```python
from build123d import *

# Parameters (mm, degrees)
BOSS_EXTRUDE1_DEPTH = 2
CUT_EXTRUDE1_DEPTH  = 10


with BuildPart() as part:
    # Sketch1 → Boss-Extrude1 (new body)
    with BuildSketch(Plane.XY):
        with BuildLine():
            Line((-26.516504294, 44.194173824), (-44.194173824, 26.516504294))
            ThreePointArc((-44.194173824, 26.516504294), (-36.270318491, 0), (-44.194173824, -26.516504294))
            Line((-44.194173824, -26.516504294), (-26.516504294, -44.194173824))
            ThreePointArc((-26.516504294, -44.194173824), (0, -36.270318491), (26.516504294, -44.194173824))
            Line((26.516504294, -44.194173824), (44.194173824, -26.516504294))
            ThreePointArc((44.194173824, -26.516504294), (36.270318491, 0), (44.194173824, 26.516504294))
            Line((44.194173824, 26.516504294), (26.516504294, 44.194173824))
            ThreePointArc((26.516504294, 44.194173824), (0, 36.270318491), (-26.516504294, 44.194173824))
        make_face()
    extrude(amount=BOSS_EXTRUDE1_DEPTH)

    # Sketch2 → Cut-Extrude1 (cut)
    with BuildSketch(Plane(origin=(0, 0, 0), x_dir=(-1, 0, 0), z_dir=(0, 0, -1))):
        with BuildLine():
            Line((-27.708756501, -8.757507261), (-27.708756501, 8.757507261))
            ThreePointArc((-27.708756501, 8.757507261), (-22.708756501, 13.757507261), (-17.708756501, 8.757507261))
            Line((-17.708756501, 8.757507261), (-17.708756501, -8.757507261))
            ThreePointArc((-17.708756501, -8.757507261), (-22.708756501, -13.757507261), (-27.708756501, -8.757507261))
        make_face()
        with BuildLine():
            Line((27.708756501, -8.757507261), (27.708756501, 8.757507261))
            ThreePointArc((27.708756501, 8.757507261), (22.708756501, 13.757507261), (17.708756501, 8.757507261))
            Line((17.708756501, 8.757507261), (17.708756501, -8.757507261))
            ThreePointArc((17.708756501, -8.757507261), (22.708756501, -13.757507261), (27.708756501, -8.757507261))
        make_face()
        with BuildLine():
            Line((-10.171642348, 22.620712564), (10.171642348, 22.620712564))
            ThreePointArc((10.171642348, 22.620712564), (13.631363465, 19.160991447), (10.171642348, 15.70127033))
            Line((10.171642348, 15.70127033), (-10.171642348, 15.70127033))
            ThreePointArc((-10.171642348, 15.70127033), (-13.631363465, 19.160991447), (-10.171642348, 22.620712564))
        make_face()
        with BuildLine():
            Line((-11.993928965, 31.0398289), (11.256357494, 31.0398289))
            ThreePointArc((11.256357494, 31.0398289), (12.893791994, 29.402394399), (11.256357494, 27.764959899))
            Line((11.256357494, 27.764959899), (-11.993928965, 27.764959899))
            ThreePointArc((-11.993928965, 27.764959899), (-13.631363465, 29.402394399), (-11.993928965, 31.0398289))
        make_face()
        with BuildLine():
            Line((-10.171642348, -22.620712564), (10.171642348, -22.620712564))
            ThreePointArc((10.171642348, -22.620712564), (13.631363465, -19.160991447), (10.171642348, -15.70127033))
            Line((10.171642348, -15.70127033), (-10.171642348, -15.70127033))
            ThreePointArc((-10.171642348, -15.70127033), (-13.631363465, -19.160991447), (-10.171642348, -22.620712564))
        make_face()
        with BuildLine():
            Line((-11.993928965, -31.0398289), (11.256357494, -31.0398289))
            ThreePointArc((11.256357494, -31.0398289), (12.893791994, -29.402394399), (11.256357494, -27.764959899))
            Line((11.256357494, -27.764959899), (-11.993928965, -27.764959899))
            ThreePointArc((-11.993928965, -27.764959899), (-13.631363465, -29.402394399), (-11.993928965, -31.0398289))
        make_face()
    extrude(amount=-CUT_EXTRUDE1_DEPTH, mode=Mode.SUBTRACT)


solid = part.part
```
Source: CAD feature listing. Evaluate the final solid. Frame: model axes, mm. A direction names the side the tool comes from. Round coordinates to 2 decimals unless told otherwise and drop trailing zeros. Loops run counter-clockwise (first coordinate to the right, second up) from the corner with the lowest first, then second, coordinate; pieces in that order, holes last.
(1) Material intervals for probe 1 along Y at (x, z) = (-0.5, 1.25); probe 2 along Y at (x, z) = (-5, 1.7); probe 3 along X at (y, z) = (13, 1.8), sorted ascending.
From the geometry:
probe 1: y = -36.27 to -31.04, -27.76 to -22.62, -15.7 to 15.7, 22.62 to 27.76, 31.04 to 36.27
probe 2: y = -36.53 to -31.04, -27.76 to -22.62, -15.7 to 15.7, 22.62 to 27.76, 31.04 to 36.53
probe 3: x = -38.05 to -25.35, -20.06 to 20.06, 25.35 to 38.05
(2) Section query C-C (x = 4). Output: boundary loops of the cut face in (y, z), and give its area (3 significant figures).
From the geometry:
outline: (-36.44, 0) - (-31.04, 0) - (-31.04, 2) - (-36.44, 2) - close; (-27.76, 0) - (-22.62, 0) - (-22.62, 2) - (-27.76, 2) - close; (-15.7, 0) - (15.7, 0) - (15.7, 2) - (-15.7, 2) - close; (22.62, 0) - (27.76, 0) - (27.76, 2) - (22.62, 2) - close; (31.04, 0) - (36.44, 0) - (36.44, 2) - (31.04, 2) - close
area: 105 mm2
(3) Section query B-B (x = -7). Output: boundary loops of the cut face in (y, z), and give its area (3 significant figures).
From the geometry:
outline: (-36.78, 0) - (-31.04, 0) - (-31.04, 2) - (-36.78, 2) - close; (-27.76, 0) - (-22.62, 0) - (-22.62, 2) - (-27.76, 2) - close; (-15.7, 0) - (15.7, 0) - (15.7, 2) - (-15.7, 2) - close; (22.62, 0) - (27.76, 0) - (27.76, 2) - (22.62, 2) - close; (31.04, 0) - (36.78, 0) - (36.78, 2) - (31.04, 2) - close
area: 106 mm2
(4) Access query for faces 5 (the cylindrical face through (13.63, 29.37, 0.99)), 6 (the flat face through (-1, 1, 0)). Directions: +Z, -Z, +X, -X, +Y, -Y. A direction counts if a zero-diameter tool reaches every point of the face in a straight line with its end or side. Return the directions, or none.
From the geometry:
face 5: +Z, -Z
face 6: -Z, +X, -X, +Y, -Y
(5) Section query A-A (z = 1.15). Give the number of separate pieces and of enclosed holes in the cut face, and give its area (3 significant figures).
From the geometry:
separate pieces: 1
enclosed holes: 6
area: 5,010 mm2
(6) Contact query for flat-ended pins moving along their axis: pin 1 Ø1 at (x, z) = (-0.5, 1.5) entering from -Y; pin 2 Ø0.6 at (x, z) = (-3.5, 1) entering from +Y; pin 3 Ø1 at (y, z) = (3.5, 1.5) entering from -X. Output: stop coordinate, or through.
From the geometry:
pin 1: stops at y = -36.28
pin 2: stops at y = 36.42
pin 3: stops at x = -36.44
(7) Pull-direction query (Y, two-part tool) for faces 1 (the flat face through (0, 15.701, 1)), 2 (the flat face through (0, -27.765, 1)), 3 (the cylindrical face through (-0.39, -36.27, 0.99)), 4 (the flat face through (-35.23, 35.48, 0.99)); classes: +Y half, -Y half, draft (parallel to the pull), parting line (faces both ways), or undercut.
From the geometry:
face 1: undercut
face 2: undercut
face 3: -Y half
face 4: +Y half
(8) Section query D-D (x = -33). Output: boundary loops of the cut face in (y, z).
From the geometry:
outline: (-37.71, 0) - (37.71, 0) - (37.71, 2) - (-37.71, 2) - close
